Can you work these out from the model? Positions are in its coordinate system, mm. A direction names the side the tool comes from. Coordinates: 2 decimals unless noted, no trailing zeros. Order: outer loops, then holes, each group sorted by start corner. A loop starts at its lowest first (then second) coordinate and runs counter-clockwise, first axis right, second up. Notation, with made-up numbers: (-8.5, 64.25) -> (45.5, 64.25) arc R34 cw to (45.5, 97.25) -> close; hole circle Ø10 at (-18.5, 68). An arc over 180 degrees is marked (long way). Answer in a Markdown table with one row per item. Add a question column.
1. Will this pin go through, and if not, where does the flat tip stop? pin 1 (13 mm diameter, centred on y = 0, z = 687.5, fed in from +X).
2. We'd pull the mould along X, two halves only. Please class faces 3 (the face through (0, -15, 385)), 4 (the face through (-17.5, 0, 385)), 5 (the face through (0, -17.5, 385)), 6 (the face through (15, 0, 385)): pulls with the +X half, pulls with the -X half, needs draft (parallel to the pull), parting line crosses it, or undercut.
3. Imagine slicing it at B-B on z = 364.5. Write out the boundary of the cut face in (x, y).
4. On a 3-axis mill with a long thin cutter (end or side, diameter ignored), from which of +Z, -Z, +X, -X, +Y, -Y can I reach the whole of each face in a straight line? I mean faces 1 (the face through (0, 15, 385)), 2 (the face through (17.5, 0, 385)). Say none if no direction works.
5. If I drill on line 1 along Z through (x, y) = (16.6, 0); line 2 along Y through (x, z) = (-12, 512), over which ranges is the centre line in solid material (lowest first)? Write a range as [from, to].
6. Imagine slicing it at A-A on x = -5.5. Write out the boundary of the cut face in (y, z).
Autodesk Inventor part; units mm, degrees
ref_plane "Start plane" through (0, 0, 0) normal (0, 0, 1) x (1, 0, 0)
ref_plane "End plane" through (0, 0, 780) normal (0, 0, 1) x (1, 0, 0)
ref_plane "YZ Plane" through (0, 0, 0) normal (1, 0, 0) x (0, 1, 0)
ref_plane "Start plane" through (0, 0, 0) normal (0, 0, 1) x (1, 0, 0)
ref_plane "End plane" through (0, 0, 780) normal (0, 0, 1) x (1, 0, 0)
sketch "Sketch" plane through (0, 0, 0) normal (0, 0, 1) x (1, 0, 0)
  line L0 (-17.5, -12.5) -> (-17.5, 12.5)
  line L1 (-12.5, 17.5) -> (12.5, 17.5)
  line L2 (17.5, 12.5) -> (17.5, -12.5)
  line L3 (12.5, -17.5) -> (-12.5, -17.5)
  arc A0 (-17.5, -12.5) -> (-12.5, -17.5) centre (-12.5, -12.5) ccw
  arc A1 (-12.5, 17.5) -> (-17.5, 12.5) centre (-12.5, 12.5) ccw
  arc A2 (17.5, 12.5) -> (12.5, 17.5) centre (12.5, 12.5) ccw
  arc A3 (12.5, -17.5) -> (17.5, -12.5) centre (12.5, -12.5) ccw
  arc A4 (-12.5, 15) -> (-15, 12.5) centre (-12.5, 12.5) ccw
  line L4 (-12.5, 15) -> (12.5, 15)
  arc A5 (15, 12.5) -> (12.5, 15) centre (12.5, 12.5) ccw
  line L5 (15, 12.5) -> (15, -12.5)
  arc A6 (12.5, -15) -> (15, -12.5) centre (12.5, -12.5) ccw
  line L6 (12.5, -15) -> (-12.5, -15)
  arc A7 (-15, -12.5) -> (-12.5, -15) centre (-12.5, -12.5) ccw
  line L7 (-15, -12.5) -> (-15, 12.5)
  line L8 (0, 25.9497) -> (0, -25.9497) construction
  line L9 (-25.9497, 0) -> (25.9497, 0) construction
  dimension "d7" = 5
  dimension "d10" = 35
  dimension "d11" = 35
  dimension "d12" = 2.5
  dimension "d15" = 17.5
  dimension "d16" = 17.5
extrude "Body" add sketch "Sketch" along normal up to surface (780 mm away) from surface at 0
sketch "Sketch3" plane through (0, 0, 0) normal (0, 0, 1) x (1, 0, 0)
  line L0 (0, 0) -> (10, 0)
ref_plane "Work Plane3" through (0, 0, 0) normal (0, -1, 0) x (1, 0, 0)
sketch "Sketch4" plane through (0, 0, 0) normal (0, -1, 0) x (1, 0, 0)
  line L0 (-2, 0) -> (12, 0)
  line L1 (-2, 780) -> (12, 780)
  dimension "d18" = 780
sketch "Sketch5" plane through (-17.5, 12.5, 0) normal (-1, 0, 0) x (0, 0, 1)
  line L0 (780, -25) -> (780, 0) construction
  line L1 (0, 0) -> (780, 0) construction
  line L2 (0, -25) -> (0, 0) construction
  line L3 (0, -25) -> (780, -25) construction
  line L4 (17.5, -375) -> (17.5, 70) construction
  line L5 (762.5, 70) -> (762.5, 5) construction
  line L6 (0, -25) -> (780, -25) construction
  line L7 (92.5, -25) -> (92.5, 0) construction
  line L8 (204, -25) -> (204, 0) construction
  line L9 (687.5, -25) -> (687.5, 0) construction
  line L10 (576, -25) -> (576, 0) construction
  line L11 (576, -12.5) -> (687.5, -12.5) construction
  line L12 (92.5, -12.5) -> (204, -12.5) construction
  point P0 (0, -12.5)
  dimension "d19" = 75
  dimension "d20" = 111.5
  dimension "d21" = 75
  dimension "d22" = 111.5
hole "Hole1" at (-17.5, 0, 92.5) at (-17.5, 0, 204) at (-17.5, 0, 576) at (-17.5, 0, 687.5) direction (1, 0, 0) diameter 10 end through all
equation "\"d7\" = G_IR"
equation "\"d10\" = G_H"
equation "\"d11\" = G_W"
equation "\"d12\" = G_T"
equation "\"d15\" = 0.5 * d10"
equation "\"d16\" = 0.5 * d11"
equation "\"d3\" = G_L"
equation "\"G_W\" = 35"
equation "\"G_H\" = 35"
equation "\"G_T\" = 2.5"
equation "\"G_IR\" = 5"
equation "\"G_L\" = d18"
equation "\"G_OFFSET_START\" = 0"
equation "\"G_OFFSET_END\" = 0"
properties part number "AS 1163 - C350L0 35x35x2.5 SHS - 780" material "Steel, Mild"
Answers follow:
| question | item | result |
|---|---|---|
| 1 | pin 1 | stops at x = 17.5 |
| 2 | face 3 | undercut |
| 2 | face 4 | pulls with the -X half |
| 2 | face 5 | needs draft |
| 2 | face 6 | undercut |
| 3 | outline | (-17.5, -12.5) arc R5 ccw to (-12.5, -17.5) -> (12.5, -17.5) arc R5 ccw to (17.5, -12.5) -> (17.5, 12.5) arc R5 ccw to (12.5, 17.5) -> (-12.5, 17.5) arc R5 ccw to (-17.5, 12.5) -> close; hole (-15, -12.5) arc R2.5 ccw to (-12.5, -15) -> (12.5, -15) arc R2.5 ccw to (15, -12.5) -> (15, 12.5) arc R2.5 ccw to (12.5, 15) -> (-12.5, 15) arc R2.5 ccw to (-15, 12.5) -> close |
| 4 | face 1 | +Z, -Z |
| 4 | face 2 | +Z, -Z, +X, +Y, -Y |
| 5 | line 1 | z = [0, 87.5], [97.5, 199], [209, 571], [581, 682.5], [692.5, 780] |
| 5 | line 2 | y = [-17.5, -15], [15, 17.5] |
| 6 | outline | (-17.5, 0) -> (-15, 0) -> (-15, 780) -> (-17.5, 780) -> close; (15, 0) -> (17.5, 0) -> (17.5, 780) -> (15, 780) -> close |
